```python
from build123d import *

# Parameters (mm, degrees)
SKETCH1_R           = 37
SKETCH1_R_2         = 2
BOSS_EXTRUDE1_DEPTH = 26
SKETCH2_R           = 25
SKETCH2_R_2         = 9
CUT_EXTRUDE1_DEPTH  = 10


with BuildPart() as part:
    # Sketch1 → Boss-Extrude1 (new body)
    with BuildSketch(Plane.XY):
        with Locations(Location((0, 0, 0), (0, 0, 180))):
            Circle(SKETCH1_R)
        with Locations(Location((0, 0, 0), (0, 0, 180))):
            Circle(SKETCH1_R_2, mode=Mode.SUBTRACT)
    extrude(amount=BOSS_EXTRUDE1_DEPTH)

    # Sketch2 → Cut-Extrude1 (cut)
    with BuildSketch(Plane(origin=(0, 0, 0), x_dir=(-1, 0, 0), z_dir=(0, 0, -1))):
        Circle(SKETCH2_R)
        Circle(SKETCH2_R_2, mode=Mode.SUBTRACT)
    cut_extrude1 = extrude(amount=-CUT_EXTRUDE1_DEPTH, mode=Mode.SUBTRACT)

    # Mirror1: Cut-Extrude1 across plane
    add(cut_extrude1.mirror(Plane(origin=(0, 0, 13), x_dir=(1, 0, 0), z_dir=(0, 0, -1))), mode=Mode.SUBTRACT)


solid = part.part
```
The listing builds one solid part. Answer for the finished solid, in the listing's coordinates (mm). A direction names the side the tool comes from. Coordinates: 2 decimals unless noted, no trailing zeros. Loops run counter-clockwise (first coordinate to the right, second up) from the corner with the lowest first, then second, coordinate; pieces in that order, holes last. Notation, with made-up numbers: M -18,-16.75 L 34,-16.75 A28 cw 34,13.25 Z; hole C -14.75,-20.75 d7. An arc over 180 degrees is marked long. Answer as a JSON object with one key per item and string values. Group by question number.
Item 1: Which of the six approach directions +Z, -Z, +X, -X, +Y, -Y give full straight-line access (tool end or side, diameter ignored) to faces 1 (the face through (-23.846, 7.509, 4.93)), 2 (the face through (0, 2, 13)), 3 (the face through (1.172, 8.923, 21.07))?
Item 2: Consider L1, parallel to Y at x = 0, z = 20.75; L2, parallel to Y at x = 6, z = 7.5; L3, parallel to Y at x = 0, z = 12.5. Determine where each line is inside the solid, lowest interval first.
Item 3: Section A-A (y = 0) is taken. Write down the section's boundary in (x, z), and give its area (3 significant figures).
Item 4: Each of these flat-tipped pins is pushed along its axis until it touches: P1, Ø6, axis at y = -16.5, z = 19.5, coming from the +X side; P2, Ø5, axis at x = 29, z = 8.5, coming from the -Y side; P3, Ø8, axis at x = 17, z = 8, coming from the -Y side. Where does it stop, or does it pass through?
Item 5: Determine the mould class of faces 4 (the face through (-17.073, 32.825, 12.818)), 5 (the face through (0, -11, 16)), 6 (the face through (-2, 2, 26)) for opening direction X: +X half, -X half, draft (parallel to the pull), parting line (faces both ways), or undercut.
Item 6: Section C-C (z = 8.5) is taken. Write down the section's boundary in (x, y).
Item 7: Section D-D (x = -21) is taken. Write down the section's boundary in (y, z), and give its area (3 significant figures).
Solved:
{
 "1": {"face 1": "-Z", "face 2": "+Z, -Z", "face 3": "+Z"},
 "2": {"L1": "y = -37 to -25, -9 to -2, 2 to 9, 25 to 37", "L2": "y = -36.51 to -24.27, -6.71 to 6.71, 24.27 to 36.51", "L3": "y = -37 to -2, 2 to 37"},
 "3": {"outline": "M -37,0 L -25,0 L -25,10 L -9,10 L -9,0 L -2,0 L -2,26 L -9,26 L -9,16 L -25,16 L -25,26 L -37,26 Z; M 2,0 L 9,0 L 9,10 L 25,10 L 25,0 L 37,0 L 37,26 L 25,26 L 25,16 L 9,16 L 9,26 L 2,26 Z", "area": "1,180 mm2"},
 "4": {"P1": "stops at x = 34.45", "P2": "stops at y = -25.82", "P3": "stops at y = -34.64"},
 "5": {"face 4": "parting line", "face 5": "undercut", "face 6": "draft"},
 "6": {"outline": "C 0,0 d74; C 0,0 d18; hole C 0,0 d50; hole C 0,0 d4"},
 "7": {"outline": "M -30.46,0 L -13.56,0 L -13.56,10 L 13.56,10 L 13.56,0 L 30.46,0 L 30.46,26 L 13.56,26 L 13.56,16 L -13.56,16 L -13.56,26 L -30.46,26 Z", "area": "1,040 mm2"}
}
